Work out the finished part from the listing and answer in its coordinate system (mm). Face numbers are marked on the shaded views. Coordinates: 2 decimals unless noted, no trailing zeros. Order: outer loops, then holes, each group sorted by start corner. A loop starts at its lowest first (then second) coordinate and runs counter-clockwise, first axis right, second up. Notation, with made-up numbers: (89, -36.5) - (96, -36.5) arc R24 ccw to (96, -4.5) - close; hole circle Ø11 at (39.5, 81.5). An arc over 180 degrees is marked (long way). Answer as a JSON object with one key per item and string values. Group by question number.
1) Each of these flat-tipped pins is pushed along its axis until it touches: P1, Ø6, axis at x = 6.5, y = -5.5, coming from the +Z side; P2, Ø1.8, axis at x = -37, z = -8.5, coming from the +Y side (3 decimals); P3, Ø6.5, axis at x = -38.1, z = 0, coming from the +Y side; P4, Ø1, axis at x = -9.5, z = 12.5, coming from the -Y side. Where does it stop, or does it pass through?
2) The mould has two halves that part along X. Classify the marked faces 1 and 2: released by +X, released by -X, zero draft, split by the parting line, or undercut.
3) Section C-C (y = -11.75) is taken. Give the vertices of the cut face in (x, z) (1 decimal).
4) Section B-B (y = 5.25) is taken. Count the separate pieces of the cut face and the enclosed holes in it, plus the area to 3 significant figures.
5) Section A-A (y = -5) is taken. Give the vertices of the cut face in (x, z), plus the area to 3 significant figures.
6) Find the intervals of material crossed by line 1 along X through (y, z) = (8.5, 20); line 2 along Z through (x, y) = (19.05, 9.9); line 3 along Z through (x, y) = (31, 11.5), in increasing order.
from build123d import *

# Parameters (mm, degrees)
SKETCH1_R                                        = 45.466
BOSS_EXTRUDE1_DEPTH                              = 25.4
CSK_FOR_1_4_FLAT_HEAD_MACHINE_SCREW1_D           = 6.5278
CSK_FOR_1_4_FLAT_HEAD_MACHINE_SCREW1_DEPTH       = 25.4
CSK_FOR_1_4_FLAT_HEAD_MACHINE_SCREW1_CSINK_D     = 12.8778
CSK_FOR_1_4_FLAT_HEAD_MACHINE_SCREW1_CSINK_ANGLE = 82
CSK_FOR_1_4_FLAT_HEAD_MACHINE_SCREW1_TIP         = 1.961148974
SKETCH8_R                                        = 46.955588052
CUT_EXTRUDE2_DEPTH                               = 12.7
SKETCH4_R                                        = 2.54
CUT_EXTRUDE3_DEPTH                               = 13.7
SKETCH9_R                                        = 2.921
CUT_EXTRUDE4_DEPTH                               = 5.08
SKETCH11_R                                       = 3.302
CUT_EXTRUDE5_DEPTH                               = 13.7
CIRPATTERN2_COUNT                                = 24
CIRPATTERN3_COUNT                                = 24


with BuildPart() as part:
    # Sketch1 → Boss-Extrude1 (new body)
    with BuildSketch(Plane(origin=(0, 0, 0), x_dir=(1, 0, 0), z_dir=(0, 1, 0))):
        Circle(SKETCH1_R)
    extrude(amount=BOSS_EXTRUDE1_DEPTH)

    # CSK for 1_4 Flat Head Machine Screw1
    with Locations(Plane(origin=(0, 25.4, 0), x_dir=(1, 0, 0), z_dir=(0, 1, 0))):
        with Locations((0, 0)):
            CounterSinkHole(CSK_FOR_1_4_FLAT_HEAD_MACHINE_SCREW1_D / 2, CSK_FOR_1_4_FLAT_HEAD_MACHINE_SCREW1_CSINK_D / 2, depth=CSK_FOR_1_4_FLAT_HEAD_MACHINE_SCREW1_DEPTH, counter_sink_angle=CSK_FOR_1_4_FLAT_HEAD_MACHINE_SCREW1_CSINK_ANGLE)
            with Locations((0, 0, -(CSK_FOR_1_4_FLAT_HEAD_MACHINE_SCREW1_DEPTH + CSK_FOR_1_4_FLAT_HEAD_MACHINE_SCREW1_TIP / 2))):  # 118° drill point
                Cone(0, CSK_FOR_1_4_FLAT_HEAD_MACHINE_SCREW1_D / 2, CSK_FOR_1_4_FLAT_HEAD_MACHINE_SCREW1_TIP, mode=Mode.SUBTRACT)

    # Sketch8 → Cut-Extrude2 (cut)
    with BuildSketch(Plane(origin=(0, 25.4, 0), x_dir=(1, 0, 0), z_dir=(0, 1, 0))):
        Circle(SKETCH8_R)
    extrude(amount=-CUT_EXTRUDE2_DEPTH, mode=Mode.SUBTRACT)

    # Sketch4 → Cut-Extrude3 (cut, through all)
    with BuildSketch(Plane.XZ):
        with Locations((0, 38.1)):
            Circle(SKETCH4_R)
    cut_extrude3 = extrude(amount=-CUT_EXTRUDE3_DEPTH, mode=Mode.SUBTRACT)

    # Sketch9 → Cut-Extrude4 (cut)
    with BuildSketch(Plane(origin=(0, 12.7, 0), x_dir=(1, 0, 0), z_dir=(0, 1, 0))):
        with Locations((0, -38.1)):
            Circle(SKETCH9_R)
    cut_extrude4 = extrude(amount=-CUT_EXTRUDE4_DEPTH, mode=Mode.SUBTRACT)

    # Sketch11 → Cut-Extrude5 (cut, through all)
    with BuildSketch(Plane(origin=(0, 12.7, 0), x_dir=(1, 0, 0), z_dir=(0, 1, 0))):
        Circle(SKETCH11_R)
    extrude(amount=-CUT_EXTRUDE5_DEPTH, mode=Mode.SUBTRACT)

    # CirPattern2: Cut-Extrude3 ×24 about axis
    cirpattern2_axis = Axis((0, 0, 0), (0, 1, 0))
    for i in range(1, CIRPATTERN2_COUNT):
        add(cut_extrude3.rotate(cirpattern2_axis, i * 360 / CIRPATTERN2_COUNT), mode=Mode.SUBTRACT)

    # CirPattern3: Cut-Extrude4 ×24 about axis
    cirpattern3_axis = Axis((0, 0, 0), (0, 1, 0))
    for i in range(1, CIRPATTERN3_COUNT):
        add(cut_extrude4.rotate(cirpattern3_axis, i * 360 / CIRPATTERN3_COUNT), mode=Mode.SUBTRACT)

    # Sketch13 → Revolve1 (revolve)
    with BuildSketch(Plane.YZ):
        with BuildLine():
            Line((0, 0), (-14.179303561, 0))
            ThreePointArc((-14.179303561, 0), (-14.007568062, 1.162621435), (-13.472719499, 2.209100627))
            Line((-13.472719499, 2.209100627), (0, 19.05))
            Line((0, 19.05), (0, 0))
        make_face()
    revolve(axis=Axis((0, 0, 0), (0, -1, 0)))


solid = part.part
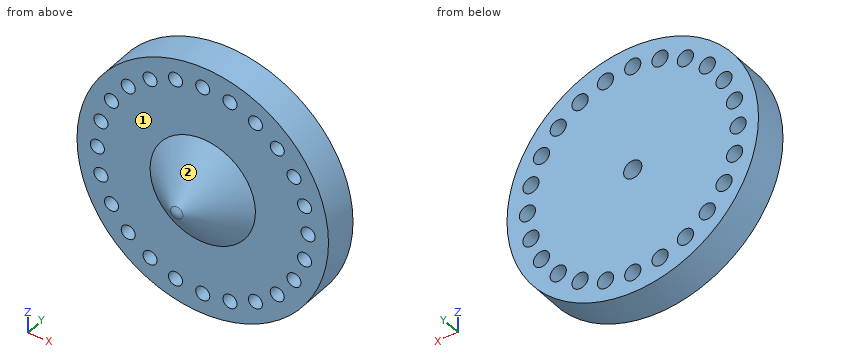
Report:
{
 "1": {"P1": "stops at z = 14.72", "P2": "passes through", "P3": "stops at y = 12.7", "P4": "stops at y = -3.08"},
 "2": {"face 1": "zero draft", "face 2": "split by the parting line"},
 "3": {"outline": "circle Ø8.7 at (0, 0)"},
 "4": {"separate pieces": "1", "enclosed holes": "25", "area": "5,970 mm²"},
 "5": {"outline": "circle Ø25.6 at (0, 0)", "area": "515 mm²"},
 "6": {"line 1": "x = -40.83 to -35.76, -30.23 to 30.23, 35.76 to 40.83", "line 2": "z = -41.28 to -35.92, -30.07 to 30.07, 35.92 to 41.28", "line 3": "z = -33.26 to -21.18, -16.92 to 16.92, 21.18 to 33.26"}
}
